Job drawing, mm, ordinate dimensions from the low corner. One solid piece. Round coordinates to 2 decimals unless told otherwise and drop trailing zeros. Order: outer loops, then holes, each group sorted by start corner. A loop starts at its lowest first (then second) coordinate and runs counter-clockwise, first axis right, second up. Notation, with made-up numbers: (56, -32.5) -> (86, -32.5) arc R18 cw to (86, -10.5) -> close; hole circle Ø11 at (-29.5, 18). An arc over 180 degrees is marked (long way). Use CSV: the item, a comma, the result in double quotes.
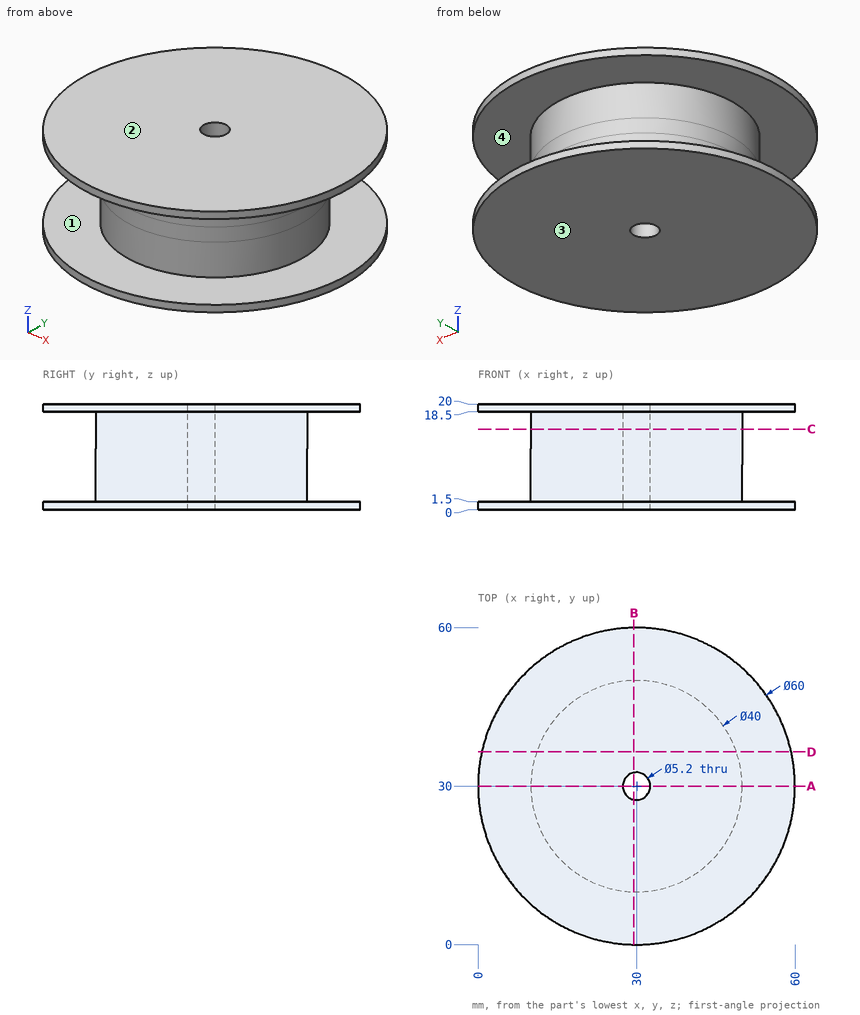
(1) Drop flat-ended pins along their axis: P1, Ø5, axis at x = 25, z = 11, coming from the +Y side; P2, Ø1.5, axis at y = 48, z = 18, coming from the -X side; P3, Ø5, axis at y = 17, z = 6, coming from the +X side. Give the stop position or say it passes through.
Reply:
P1,"y = 49.84"
P2,"x = 5.59"
P3,"x = 47.02"
(2) Probe probe 1 along Z at (x, y) = (3, 32.5); probe 2 along Y at (x, z) = (30, 8.25); probe 3 along X at (y, z) = (30.5, 6). List the from-to ranges inside material, lowest first. Write a range as [from, to].
Reply:
probe 1,"[0, 1.5], [18.5, 20]"
probe 2,"[10, 27.4], [32.6, 50]"
probe 3,"[10.01, 27.45], [32.55, 49.99]"
(3) Pull direction Z, two halves, no side cores. Call the marked faces 1, 2, 3 and 4: released by +Z, released by -Z, zero draft, split by the parting line, or undercut.
Reply:
face 1,"undercut"
face 2,"released by +Z"
face 3,"released by -Z"
face 4,"undercut"
(4) Cut at D-D, the plane y = 36.5. Give the cut face in (x, z).
Reply:
outline,"(0.71, 0) -> (59.29, 0) -> (59.29, 1.5) -> (48.91, 1.5) -> (48.91, 18.5) -> (59.29, 18.5) -> (59.29, 20) -> (0.71, 20) -> (0.71, 18.5) -> (11.09, 18.5) -> (11.09, 1.5) -> (0.71, 1.5) -> close"
(5) Cut at B-B, the plane x = 29.5. Give the cut face in (y, z), then the cut area to 3 significant figures.
Reply:
outline,"(0, 0) -> (27.45, 0) -> (27.45, 20) -> (0, 20) -> (0, 18.5) -> (10.01, 18.5) -> (10.01, 1.5) -> (0, 1.5) -> close; (32.55, 0) -> (60, 0) -> (60, 1.5) -> (49.99, 1.5) -> (49.99, 18.5) -> (60, 18.5) -> (60, 20) -> (32.55, 20) -> close"
area,"758 mm2"
(6) Cut at A-A, the plane y = 30. Give the cut face in (x, z).
Reply:
outline,"(0, 0) -> (27.4, 0) -> (27.4, 20) -> (0, 20) -> (0, 18.5) -> (10, 18.5) -> (10, 1.5) -> (0, 1.5) -> close; (32.6, 0) -> (60, 0) -> (60, 1.5) -> (50, 1.5) -> (50, 18.5) -> (60, 18.5) -> (60, 20) -> (32.6, 20) -> close"
(7) Cut at C-C, the plane z = 15.25. Give the cut face in (x, y).
Reply:
outline,"circle Ø40 at (30, 30); hole circle Ø5.2 at (30, 30)"
